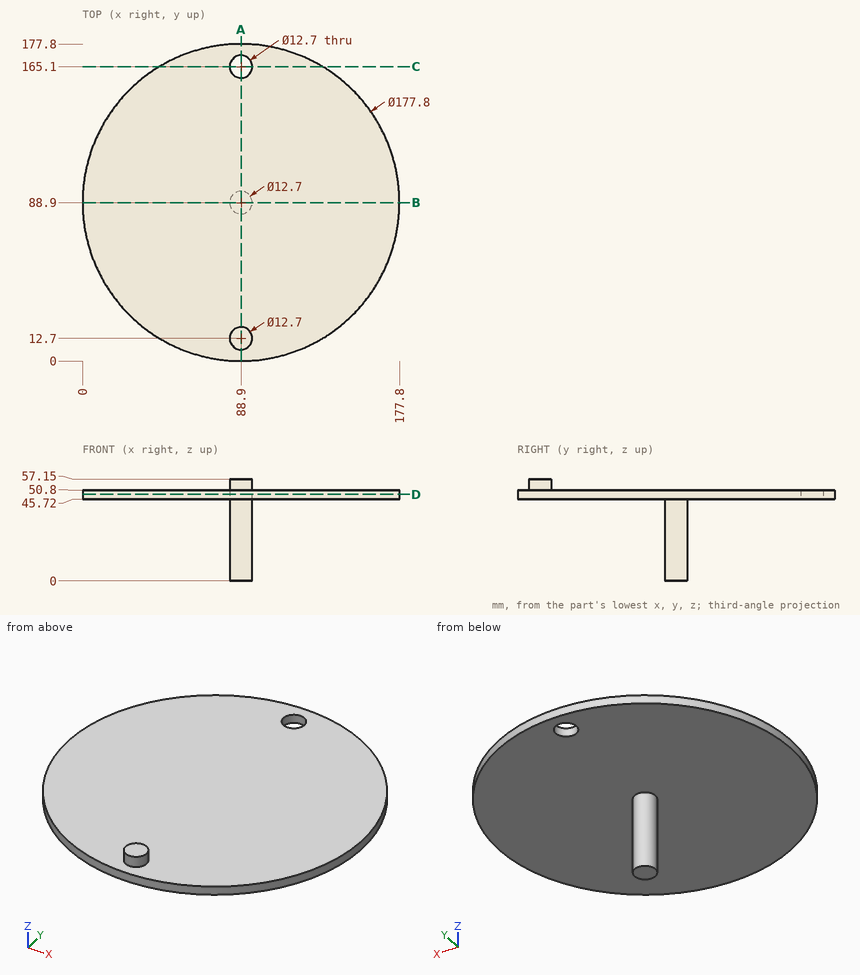
Geometry check sheet. Reference: drawing and pictorial views, mm from the part's lowest x, y, z. Give positions to 0.01 mm unless a question says otherwise; leave off trailing zeros. Order: outer loops, then holes, each group sorted by start corner. A loop starts at its lowest first (then second) coordinate and runs counter-clockwise, first axis right, second up. Notation, with made-up numbers: M 10,-4 L 57,-4 A28 ccw 57,17 Z; hole C -16.5,17.25 d10. An arc over 180 degrees is marked long. Answer in a Markdown table with one row per item. Add a question column.
Q1. Sectioned sample at A-A, the plane x = 88.9. Record the boundary of the cut face in (y, z).
Q2. Thickness scan on L1, parallel to Y at x = 88.9, z = 47.5; L2, parallel to Z at x = 37, y = 58.5; L3, parallel to X at y = 165, z = 47. Record the ranges inside material, lowest first.
Q3. Gauge pin test, flat ends, axial feed: pin 1 Ø1.5 at (x, y) = (67.5, 82.5) entering from +Z; pin 2 Ø20.5 at (x, y) = (88.9, 165.1) entering from -Z. Record the tip position at first contact, or that the pin passes through.
Q4. Sectioned sample at D-D, the plane z = 48.5. Record the boundary of the cut face in (x, y).
Q5. Sectioned sample at B-B, the plane y = 88.9. Record the boundary of the cut face in (x, z), and give its area (3 significant figures).
Q6. Sectioned sample at C-C, the plane y = 165.1. Record the boundary of the cut face in (x, z), and give its area (3 significant figures).
Verdict:
| question | item | result |
|---|---|---|
| 1 | outline | M 0,45.72 L 82.55,45.72 L 82.55,0 L 95.25,0 L 95.25,45.72 L 158.75,45.72 L 158.75,50.8 L 19.05,50.8 L 19.05,57.15 L 6.35,57.15 L 6.35,50.8 L 0,50.8 Z; M 171.45,45.72 L 177.8,45.72 L 177.8,50.8 L 171.45,50.8 Z |
| 2 | L1 | 0 to 158.75, 171.45 to 177.8 |
| 2 | L2 | 45.72 to 50.8 |
| 2 | L3 | 42.94 to 82.55, 95.25 to 134.86 |
| 3 | pin 1 | z = 50.8 |
| 3 | pin 2 | z = 45.72 |
| 4 | outline | C 88.9,88.9 d177.8; hole C 88.9,165.1 d12.7 |
| 5 | outline | M 0,45.72 L 82.55,45.72 L 82.55,0 L 95.25,0 L 95.25,45.72 L 177.8,45.72 L 177.8,50.8 L 0,50.8 Z |
| 5 | area | 1,480 mm² |
| 6 | outline | M 43.11,45.72 L 82.55,45.72 L 82.55,50.8 L 43.11,50.8 Z; M 95.25,45.72 L 134.69,45.72 L 134.69,50.8 L 95.25,50.8 Z |
| 6 | area | 401 mm² |
